Geometry check sheet. Reference: the model listing, model coordinates, mm. Face numbers are marked on the shaded views. A direction names the side the tool comes from. Round coordinates to 2 decimals unless told otherwise and drop trailing zeros. Write each loop counter-clockwise with the first axis right and the second up, starting at its lowest first coordinate (ties: lowest second). Pieces come first, ordered by that corner, then holes. Notation, with made-up numbers: M -8,52.25 L 28,52.25 A25 ccw 28,78.25 Z; hole C -39,26 d9. An arc over 180 degrees is marked long. Use a Markdown table: item, result.
Autodesk Inventor part; units mm, degrees
ref_plane "Plano de trabajo1" through (0, 5, -50) normal (1, 0, 0) x (0, 0, -1)
ref_plane "Plano de trabajo2" through (0, 15, 0) normal (0, -1, 0) x (1, 0, 0)
ref_plane "YZ Plane" through (0, 0, 0) normal (1, 0, 0) x (0, 1, 0)
sketch "Boceto1" plane through (0, 0, 0) normal (0, 1, 0) x (-1, 0, 0)
  line L0 (27.5, 50) -> (-27.5, 50)
  line L1 (-27.5, 50) -> (-27.5, -50)
  line L2 (-27.5, -50) -> (27.5, -50)
  line L3 (27.5, -50) -> (27.5, 50)
  line L4 (27.5, 50) -> (-27.5, -50) construction
  line L5 (-27.5, 50) -> (27.5, -50) construction
  point P0 (0, 0)
  dimension "d0" = 55
  dimension "d1" = 100
extrude "Extrusión1" add sketch "Boceto1" along normal blind 30
sketch "Boceto2" plane through (27.5, 0, -50) normal (0, 0, -1) x (-1, 0, 0)
  line L0 (22.5, 25) -> (32.5, 25)
  line L1 (32.5, 25) -> (32.5, 5)
  line L2 (32.5, 5) -> (22.5, 5)
  line L3 (22.5, 5) -> (22.5, 25)
  line L4 (22.5, 25) -> (32.5, 5) construction
  line L5 (32.5, 25) -> (22.5, 5) construction
  line L6 (0, 30) -> (55, 30)
  line L7 (0, 0) -> (0, 30)
  line L8 (55, 0) -> (55, 30)
  point P0 (27.5, 0)
  point P1 (27.5, 15)
  point P2 (27.5, 25)
  dimension "d4" = 10
  dimension "d5" = 20
  dimension "d6" = 5
  dimension "d7" = 22.5
  dimension "d24" = 22.5
extrude "Extrusión2" add sketch "Boceto2" along normal blind 10
sketch "Boceto3" plane through (-27.5, 0, 50) normal (0, 0, 1) x (1, 0, 0)
  circle A0 centre (27.5, 20) radius 5
  line L0 (0, 30) -> (55, 30)
  point P0 (27.5, 0)
  point P1 (27.5, 30)
  dimension "d10" = 10
  dimension "d11" = 10
extrude "Extrusión3" cut sketch "Boceto3" against normal blind 15
sketch "Boceto4" plane through (0, 30, 0) normal (0, 1, 0) x (1, 0, 0)
  line L0 (-20, 23) -> (20, 23)
  line L1 (20, 23) -> (20, -23)
  line L2 (20, -23) -> (-20, -23)
  line L3 (-20, -23) -> (-20, 23)
  line L4 (-20, 23) -> (20, -23) construction
  line L5 (20, 23) -> (-20, -23) construction
  point P0 (0, 0)
  dimension "d14" = 40
  dimension "d15" = 46
extrude "Extrusión4" cut sketch "Boceto4" against normal blind 20
ref_plane "Plano de trabajo1" through (0, 5, -50) normal (1, 0, 0) x (0, 0, -1)
sketch "Boceto5" plane through (0, 5, -50) normal (1, 0, 0) x (0, 0, -1)
  line L0 (7.5, 0) -> (0, -2.5)
  line L1 (0, -2.5) -> (0, 0)
  line L2 (0, 0) -> (7.5, 0)
  point P0 (-50, -5)
  point P1 (0, -5)
  point P2 (10, 0)
  dimension "d25" = 2.5
  dimension "d26" = 2.5
extrude "Extrusión5" add sketch "Boceto5" along normal mid plane 8
ref_plane "Plano de trabajo2" through (0, 15, 0) normal (0, -1, 0) x (1, 0, 0)
sketch "Boceto6" plane through (0, 15, 0) normal (0, -1, 0) x (1, 0, 0)
  line L0 (5, -50) -> (8, -50)
  line L1 (27.5, -50) -> (-27.5, -50)
  line L2 (5, -57) -> (8, -50)
  line L3 (4, -50) -> (5, -50)
  line L4 (5, -50) -> (5, -57)
  line L5 (0, -50.2371) -> (0, -56.5746)
  line L6 (-5, -50) -> (-8, -50)
  line L7 (-27.5, -50) -> (27.5, -50)
  line L8 (-5, -57) -> (-8, -50)
  line L9 (-4, -50) -> (-5, -50)
  line L10 (-5, -50) -> (-5, -57)
  point P0 (0, 0)
  point P1 (5, -60)
  point P2 (-5, -60)
  dimension "d29" = 3
  dimension "d30" = 3
extrude "Extrusión6" add sketch "Boceto6" along normal mid plane 8
sketch "Boceto7" plane through (27.5, 0, 50) normal (1, 0, 0) x (0, 0, -1)
  point P0 (50, 0)
ref_plane "Plano de trabajo4" through (-20, 30, -23) normal (0, 0, 1) x (1, 0, 0)
sketch "Boceto8" plane through (27.5, 0, 50) normal (1, 0, 0) x (0, 0, -1)
  line L0 (58, 22) -> (88, 22)
  circle A0 centre (83, 17) radius 1.75
  line L1 (63, 17) -> (83, 17)
  line L2 (88, 22) -> (88, 12)
  circle A1 centre (63, 17) radius 1.75
  line L3 (58, 12) -> (88, 22) construction
  line L4 (58, 22) -> (88, 12) construction
  line L5 (58, 12) -> (58, 22)
  line L6 (88, 12) -> (58, 12)
  line L7 (73, 30) -> (73, 10)
  line L8 (0, 30) -> (100, 30)
  point P0 (50, 0)
  point P1 (72.9522, 12.5553)
  point P2 (57.9522, 14.5161)
  point P3 (72.9522, 12.5553)
  point P4 (88, 17)
  dimension "d34" = 10
  dimension "d35" = 30
  dimension "d36" = 5
  dimension "d37" = 5
  dimension "d38" = 5
  dimension "d39" = 5
  dimension "d40" = 10
  dimension "d41" = 8
hole "Agujero1" at (27.5, 17, -13) at (27.5, 17, -33) direction (-1, 0, 0) diameter 3.5 end through all
split "Dividir1" plane through (-20, 30, -23) removes the side toward (0, 0, 1)
properties part number "camera_support_2_1"
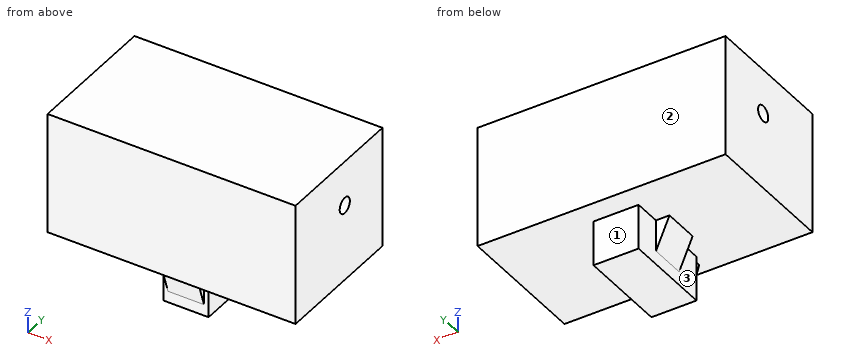
Item 1: Cross-section at B-B, the plane x = -12.5. Record the cut outline in (y, z), and give its area (3 significant figures).
Outcome:
| item | result |
|---|---|
| outline | M 0,-50 L 30,-50 L 30,-23 L 0,-23 Z; hole C 17,-33 d3.5 |
| area | 800 mm2 |
Item 2: Cross-section at C-C, the plane y = 17. Record the cut outline in (x, z), and give its area (3 significant figures).
Outcome:
| item | result |
|---|---|
| outline | M -27.5,-50 L -8,-50 L -5,-57 L -5,-60 L 5,-60 L 5,-57 L 8,-50 L 27.5,-50 L 27.5,-34.75 L -27.5,-34.75 Z; M -27.5,-31.25 L 27.5,-31.25 L 27.5,-23 L -27.5,-23 Z |
| area | 1,410 mm2 |
Item 3: Cross-section at D-D, the plane z = -56. Record the cut outline in (x, y), and give its area (3 significant figures).
Outcome:
| item | result |
|---|---|
| outline | M -5.43,11 L -5,11 L -5,5 L -4,5 L -4,4.5 L 4,4.5 L 4,5 L 5,5 L 5,11 L 5.43,11 L 5.43,19 L 5,19 L 5,25 L -5,25 L -5,19 L -5.43,19 Z |
| area | 211 mm2 |
Item 4: Cross-section at A-A, the plane z = -33. Record the cut outline in (x, y), and give its area (3 significant figures).
Outcome:
| item | result |
|---|---|
| outline | M -27.5,0 L 27.5,0 L 27.5,15.25 L -27.5,15.25 Z; M -27.5,18.75 L 27.5,18.75 L 27.5,30 L -27.5,30 Z |
| area | 1,460 mm2 |
Item 5: Material ranges on line 1 along Y through (x, z) = (9.5, -33); line 2 along Z through (x, y) = (3.5, 17); line 3 along Z through (x, y) = (15, 24), recorded low to high. Write a range as from..to.
Outcome:
| item | result |
|---|---|
| line 1 | y = 0..15.25, 18.75..30 |
| line 2 | z = -60..-34.75, -31.25..-23 |
| line 3 | z = -50..-23 |
Item 6: Access from +Z, -Z, +X, -X, +Y, -Y to the whole of each face (thin tool, end or side, straight path). Record for the marked faces 1, 2 and 3.
Outcome:
| item | result |
|---|---|
| face 1 | -Z, +X, -X, +Y |
| face 2 | +Z, -Z, +X, -X, +Y |
| face 3 | -Z, -X |
Item 7: Go/stop test with flat-tipped pins: pin 1 (0.9 mm diameter, centred on x = 6.5, z = -54.5, fed in from -Y); pin 2 (8 mm diameter, centred on y = 13, z = -55.5, fed in from -X); pin 3 (8 mm diameter, centred on x = 1, z = -55.5, fed in from -Y); pin 4 (2 mm diameter, centred on x = -21, z = -52.5, fed in from -Y). Record where each tip stops, or that it passes through.
Outcome:
| item | result |
|---|---|
| pin 1 | stops at y = 11 |
| pin 2 | stops at x = -7.36 |
| pin 3 | stops at y = 3 |
| pin 4 | passes through |
